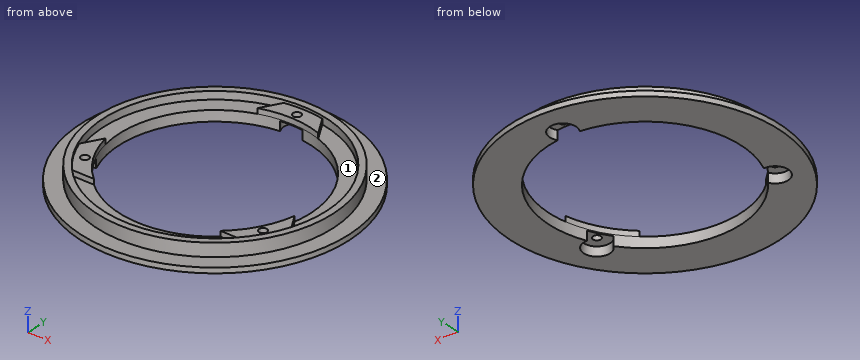
```python
from build123d import *

# Parameters (mm, degrees)
SKETCH_R          = 51
SKETCH_R_2        = 36.5
PAD_DEPTH         = 2
SKETCH001_R       = 45
SKETCH001_R_2     = 42.5
PAD001_DEPTH      = 5
SKETCH002_R       = 43
SKETCH002_R_2     = 36.5
PAD002_DEPTH      = 2
SKETCH004_R       = 5
POCKET001_DEPTH   = 3.5
PAD003_DEPTH      = 2
SKETCH003_R       = 1.5
POCKET_DEPTH      = 4.001
POCKET_DEPTH_BACK = 3.001


with BuildPart() as part:
    # Sketch → Pad (new body)
    with BuildSketch(Plane.XY):
        Circle(SKETCH_R)
        Circle(SKETCH_R_2, mode=Mode.SUBTRACT)
    extrude(amount=PAD_DEPTH)

    # Sketch001 (on Face4 of Pad) → Pad001 (join)
    with BuildSketch(Plane.XY.offset(2)):
        Circle(SKETCH001_R)
        Circle(SKETCH001_R_2, mode=Mode.SUBTRACT)
    extrude(amount=PAD001_DEPTH)

    # Sketch002 (on Face6 of Pad001) → Pad002 (join)
    with BuildSketch(Plane.XY.offset(2)):
        Circle(SKETCH002_R)
        Circle(SKETCH002_R_2, mode=Mode.SUBTRACT)
    extrude(amount=PAD002_DEPTH)

    # Sketch004 → Pocket001 (cut)
    with BuildSketch(Plane(origin=(0, 0, 0), x_dir=(1, 0, 0), z_dir=(0, 0, -1))):
        with Locations((33.7749907476, 19.5)):
            Circle(SKETCH004_R)
        with Locations((-33.7749907476, 19.5)):
            Circle(SKETCH004_R)
        with Locations((0, -39)):
            Circle(SKETCH004_R)
    extrude(amount=-POCKET001_DEPTH, mode=Mode.SUBTRACT)

    # Sketch005 (on Face19 of Pocket001) → Pad003 (join)
    with BuildSketch(Plane.XY.offset(4)):
        with BuildLine():
            ThreePointArc((11.5051886068, 34.6392932249), (-0.0001407701, 36.4999999997), (-11.5054557942, 34.6392044794))
            Line((-7.2870367194, 41.8706233038), (-11.5054557942, 34.6392044794))
            ThreePointArc((7.2867818781, 41.8706676548), (-0.0001293359, 42.4999999998), (-7.2870367194, 41.8706233038))
            Line((11.5051886068, 34.6392932249), (7.2867818781, 41.8706676548))
        make_face()
        with BuildLine():
            ThreePointArc((-40.0341199475, -14.2660169643), (-36.8189826795, -21.2276356301), (-32.4052284347, -27.4982030339))
            Line((-32.4052284347, -27.4982030339), (-24.0020588681, -27.4982030339))
            ThreePointArc((-35.8157008728, -7.0345981399), (-31.6106133509, -18.2488115663), (-24.0020588681, -27.4982030339))
            Line((-35.8157008728, -7.0345981399), (-40.0341199475, -14.2660169643))
        make_face()
        with BuildLine():
            Line((40.0340730114, -14.2661486785), (35.8156662827, -7.0347742486))
            ThreePointArc((24.0020588681, -27.4982030339), (31.6105684853, -18.2488892822), (35.8156662827, -7.0347742486))
            Line((24.0020588681, -27.4982030339), (32.4052284347, -27.4982030339))
            ThreePointArc((32.4052284347, -27.4982030339), (36.8189477595, -21.2276961982), (40.0340730114, -14.2661486785))
        make_face()
    extrude(amount=PAD003_DEPTH)

    # Sketch003 (on Face8 of Pad002) → Pocket (cut, two sides)
    with BuildSketch(Plane.XY.offset(4)) as pocket_sk:
        with Locations((0, 39)):
            Circle(SKETCH003_R)
        with Locations((33.7749907476, -19.5)):
            Circle(SKETCH003_R)
        with Locations((-33.7749907476, -19.5)):
            Circle(SKETCH003_R)
    extrude(amount=-POCKET_DEPTH, mode=Mode.SUBTRACT)
    extrude(pocket_sk.sketch, amount=POCKET_DEPTH_BACK, mode=Mode.SUBTRACT)


solid = part.part
```
Model file for the job. Use its own axes, mm. Face numbers are marked on the shaded views. Round coordinates to 2 decimals unless told otherwise and drop trailing zeros. Write each loop counter-clockwise with the first axis right and the second up, starting at its lowest first coordinate (ties: lowest second). Pieces come first, ordered by that corner, then holes. Notation, with made-up numbers: (11.25, 30.25) -> (18.25, 30.25) arc R16 ccw to (18.25, 54.25) -> close; hole circle Ø2 at (-0.5, 37). An arc over 180 degrees is marked (long way). Answer as CSV lines item,"result".
1. Slice it at C-C, the plane x = 31. List the corners of the cut face in (y, z), plus the area to 3 significant figures.
Resolved:
outline,"(-40.5, 0) -> (-23.66, 0) -> (-23.66, 3.5) -> (-19.27, 3.5) -> (-19.27, 6) -> (-27.5, 6) -> (-27.5, 4) -> (-29.07, 4) -> (-29.07, 7) -> (-32.62, 7) -> (-32.62, 2) -> (-40.5, 2) -> close; (19.27, 0) -> (40.5, 0) -> (40.5, 2) -> (32.62, 2) -> (32.62, 7) -> (29.07, 7) -> (29.07, 4) -> (19.27, 4) -> close"
area,"161 mm²"
2. Mould opens along X. For the marked faces 1 and 2 say: +X half, -X half, draft (parallel to the pull), parting line (faces both ways), or undercut.
Resolved:
face 1,"undercut"
face 2,"draft"
3. Pin check, flat tips, straight feed: pin 1 Ø2.5 at (x, y) = (4.5, 38.5) entering from +Z; pin 2 Ø4.5 at (x, y) = (-0.5, -38) entering from +Z; pin 3 Ø2 at (x, z) = (36.5, 2.5) entering from +Y. Stop position of each tip, or through.
Resolved:
pin 1,"z = 6"
pin 2,"z = 4"
pin 3,"y = 36.49"
4. Slice it at D-D, the plane y = -19.5. List the corners of the cut face in (x, z) (1 decimal), plus the area to 3 significant figures.
Resolved:
outline,"(-47.1, 0) -> (-38.8, 0) -> (-38.8, 3.5) -> (-35.3, 3.5) -> (-35.3, 6) -> (-37.8, 6) -> (-37.8, 7) -> (-40.6, 7) -> (-40.6, 2) -> (-47.1, 2) -> close; (-32.3, 3.5) -> (-30.9, 3.5) -> (-30.9, 6) -> (-32.3, 6) -> close; (30.9, 3.5) -> (32.3, 3.5) -> (32.3, 6) -> (30.9, 6) -> close; (35.3, 3.5) -> (38.8, 3.5) -> (38.8, 0) -> (47.1, 0) -> (47.1, 2) -> (40.6, 2) -> (40.6, 7) -> (37.8, 7) -> (37.8, 6) -> (35.3, 6) -> close"
area,"77.8 mm²"
5. Slice it at A-A, the plane x = 0. List the corners of the cut face in (y, z).
Resolved:
outline,"(-51, 0) -> (-36.5, 0) -> (-36.5, 4) -> (-42.5, 4) -> (-42.5, 7) -> (-45, 7) -> (-45, 2) -> (-51, 2) -> close; (36.5, 3.5) -> (37.5, 3.5) -> (37.5, 6) -> (36.5, 6) -> close; (40.5, 3.5) -> (44, 3.5) -> (44, 0) -> (51, 0) -> (51, 2) -> (45, 2) -> (45, 7) -> (42.5, 7) -> (42.5, 6) -> (40.5, 6) -> close"
6. Drill centre lines: line 1 (X direction, y = -19.5, z = 4.5) (1 decimal); line 2 (Y direction, x = 0, z = 4.7); line 3 (X direction, y = 38, z = 5.75). Where is each one in solid material? Low to high.
Resolved:
line 1,"-40.6 to -35.3, -32.3 to -30.9, 30.9 to 32.3, 35.3 to 40.6"
line 2,"-45 to -42.5, 36.5 to 37.5, 40.5 to 45"
line 3,"-24.1 to -19.03, -9.54 to -1.12, 1.12 to 9.54, 19.03 to 24.1"
7. Slice it at B-B, the plane y = 0. List the corners of the cut face in (x, z).
Resolved:
outline,"(-51, 0) -> (-36.5, 0) -> (-36.5, 4) -> (-42.5, 4) -> (-42.5, 7) -> (-45, 7) -> (-45, 2) -> (-51, 2) -> close; (36.5, 0) -> (51, 0) -> (51, 2) -> (45, 2) -> (45, 7) -> (42.5, 7) -> (42.5, 4) -> (36.5, 4) -> close"
